Verification items for this drawing (mm, ordinates from the low corner). Coordinates: 2 decimals unless noted, no trailing zeros. Order: outer loops, then holes, each group sorted by start corner. A loop starts at its lowest first (then second) coordinate and runs counter-clockwise, first axis right, second up.
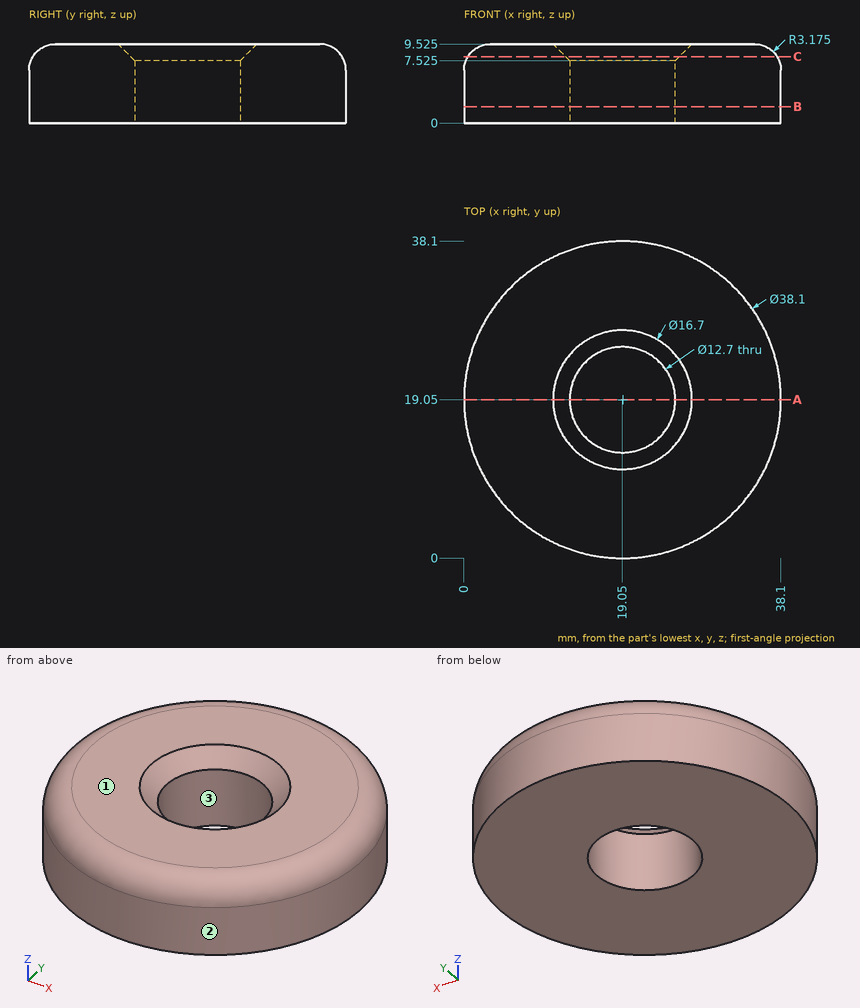
(1) Cross-section at A-A (y = 19.05). Enter the section's corners in (x, z) (3 decimals), and give its area (3 significant figures).
Filled in:
outline: (0, 0) - (12.7, 0) - (12.7, 7.525) - (10.7, 9.525) - (3.175, 9.525) arc R3.175 ccw to (0, 6.35) - close; (25.4, 0) - (38.1, 0) - (38.1, 6.35) arc R3.175 ccw to (34.925, 9.525) - (27.4, 9.525) - (25.4, 7.525) - close
area: 234 mm2
(2) Thickness scan on probe 1 along Y at (x, z) = (19.05, 2.5); probe 2 along Y at (x, z) = (23, 6); probe 3 along X at (y, z) = (23, 7.5). Record the ranges inside material, lowest first.
Filled in:
probe 1: y = 0 to 12.7, 25.4 to 38.1
probe 2: y = 0.41 to 14.08, 24.02 to 37.69
probe 3: x = 0.63 to 14.08, 24.02 to 37.47
(3) Go/stop test with flat-tipped pins: P1, Ø2, axis at x = 23.5, z = 2.5, coming from the +Y side (3 decimals); P2, Ø11.5, axis at x = 19.05, y = 19.05, coming from the +Z side; P3, Ø4, axis at x = 9.5, z = 1.5, coming from the +Y side. Record where each tip stops, or that it passes through.
Filled in:
P1: stops at y = 37.785
P2: passes through
P3: stops at y = 36.54
(4) Cross-section at C-C (z = 8). Enter the section's corners in (x, y) (3 decimals).
Filled in:
outline: circle Ø37.175 at (19.05, 19.05); hole circle Ø13.65 at (19.05, 19.05)
(5) Release check for a two-part mould opening along X. For the marked faces 1, 2 and 3 record: +X half, -X half, draft (parallel to the pull), parting line (faces both ways), or undercut.
Filled in:
face 1: draft
face 2: parting line
face 3: undercut
(6) Cross-section at B-B (z = 2). Enter the section's corners in (x, y), and give its area (3 significant figures).
Filled in:
outline: circle Ø38.1 at (19.05, 19.05); hole circle Ø12.7 at (19.05, 19.05)
area: 1,010 mm2
